Model file for the job. Use its own axes, mm. Face numbers are marked on the shaded views. A direction names the side the tool comes from. Round coordinates to 2 decimals unless told otherwise and drop trailing zeros. Loops run counter-clockwise (first coordinate to the right, second up) from the corner with the lowest first, then second, coordinate; pieces in that order, holes last. Notation, with made-up numbers: M 46,67 L 66,67 A28 cw 66,103 Z; hole C 80.5,11 d10. An arc over 180 degrees is marked long. Use a Markdown table: item, result. Add a question column.
Q1. Cut at B-B (z = -152). Give the cut face in (x, y), plus the area to 4 significant figures.
Q2. Pin check, flat tips, straight feed: pin 1 (1.9 mm diameter, centred on x = -305, z = -608, fed in from +Y); pin 2 (9 mm diameter, centred on x = -76, y = 69, fed in from -Z); pin 3 (3 mm diameter, centred on x = 179, z = -605.5, fed in from +Y); pin 4 (9 mm diameter, centred on x = 260, y = 233, fed in from +Z). Stop position of each tip, or through.
Q3. Probe line 1 (X direction, y = 49, z = -402); line 2 (Y direction, x = -209.5, z = -435); line 3 (Y direction, x = 66.5, z = -34). List the from-to ranges inside material, lowest first. Write a range as from..to.
Q4. Tool access for the marked faces 1 and 2: list every direction of +Z, -Z, +X, -X, +Y, -Y with a clear straight run to the whole face (end or side of a thin tool).
Q5. Cut at A-A (y = 185). Give the cut face in (x, z), plus the area to 3 significant figures.
Q6. Cut at C-C (x = 105). Give the cut face in (y, z).
Q7. Cut at D-D (z = -446). Give the cut face in (x, y).
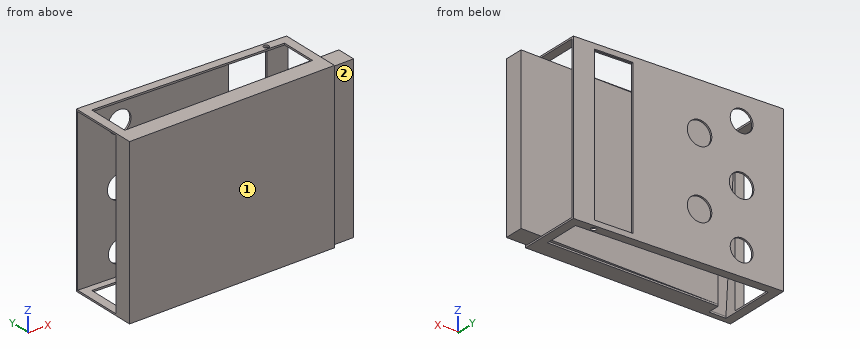
from build123d import *

# Parameters (mm, degrees)
BOSS_EXTRUDE1_DEPTH = 609.6
SHELL1_T            = -6.35
CUT_EXTRUDE1_DEPTH  = 609.6
BOSS_EXTRUDE3_DEPTH = 596.9
BOSS_EXTRUDE4_DEPTH = 95.25
SKETCH8_W           = 31.75
SKETCH8_H           = 44.45
BOSS_EXTRUDE5_DEPTH = 603.25
SKETCH9_W           = 63.5
SKETCH9_H           = 44.45
CUT_EXTRUDE2_DEPTH  = 6.35
SKETCH10_R          = 41.275
SKETCH10_R_2        = 44.45
CUT_EXTRUDE3_DEPTH  = 6.35
SKETCH12_W          = 139.7
SKETCH12_H          = 571.5
CUT_EXTRUDE4_DEPTH  = 6.35
SKETCH13_R          = 9.525
CUT_EXTRUDE5_DEPTH  = 609.6


with BuildPart() as part:
    # Sketch1 → Boss-Extrude1 (new body)
    with BuildSketch(Plane.XY):
        Polygon((-373.981578947, 0), (388.018421053, 0), (388.018421053, 228.6), (-373.981578947, 254), align=None)
    extrude(amount=-BOSS_EXTRUDE1_DEPTH)

    # Shell1
    shell1_openings = [part.faces().sort_by_distance(p)[0] for p in [
        (-373.981578947, 127, -304.8),
        (388.018421053, 114.3, -304.8),
    ]]
    offset(amount=SHELL1_T, openings=shell1_openings, kind=Kind.INTERSECTION)

    # Sketch2 → Cut-Extrude1 (cut)
    with BuildSketch(Plane.XY):
        Polygon((-342.231578947, 221.174032675), (356.268421053, 197.890699341), (356.268421053, 63.5), (-342.231578947, 63.5), align=None)
    extrude(amount=-CUT_EXTRUDE1_DEPTH, mode=Mode.SUBTRACT)

    # Sketch5 → Boss-Extrude3 (add)
    with BuildSketch(Plane.XY.offset(-603.25)):
        Polygon((-278.731578947, 63.5), (464.218421053, 76.696522884), (464.218421053, 6.35), (-278.731578947, 6.35), align=None)
    extrude(amount=BOSS_EXTRUDE3_DEPTH)

    # Sketch6 → Boss-Extrude4 (add)
    with BuildSketch(Plane.ZY.offset(278.731578947)):
        Polygon((-6.35, 63.5), (-603.25, 19.05), (-603.25, 6.35), (-6.35, 6.35), align=None)
    extrude(amount=BOSS_EXTRUDE4_DEPTH)

    # Sketch8 → Boss-Extrude5 (add)
    with BuildSketch(Plane(origin=(0, 0, -609.6), x_dir=(-1, 0, 0), z_dir=(0, 0, -1))):
        with Locations((358.106578947, 41.275)):
            Rectangle(SKETCH8_W, SKETCH8_H)
    extrude(amount=-BOSS_EXTRUDE5_DEPTH)

    # Sketch9 → Cut-Extrude2 (cut)
    with BuildSketch(Plane(origin=(0, 0, -609.6), x_dir=(-1, 0, 0), z_dir=(0, 0, -1))):
        with Locations((310.481578947, 41.275)):
            Rectangle(SKETCH9_W, SKETCH9_H)
    extrude(amount=-CUT_EXTRUDE2_DEPTH, mode=Mode.SUBTRACT)

    # Sketch10 → Cut-Extrude3 (cut)
    with BuildSketch(Plane(origin=(8.042195806, 241.265874175, 0), x_dir=(0.999444907, -0.03331483, 0), z_dir=(0.03331483, 0.999444907, 0))):
        with Locations((-229.835951262, 88.9)):
            Circle(SKETCH10_R)
        with Locations((-229.835951262, 520.7)):
            Circle(SKETCH10_R)
        with Locations((-77.435951262, 431.8)):
            Circle(SKETCH10_R_2)
        with Locations((-77.435951262, 177.8)):
            Circle(SKETCH10_R_2)
        with Locations((-229.835951262, 304.8)):
            Circle(SKETCH10_R_2)
    extrude(amount=-CUT_EXTRUDE3_DEPTH, mode=Mode.SUBTRACT)

    # Sketch12 → Cut-Extrude4 (cut)
    with BuildSketch(Plane(origin=(8.042195806, 241.265874175, 0), x_dir=(0.999444907, -0.03331483, 0), z_dir=(0.03331483, 0.999444907, 0))):
        with Locations((234.137264544, 304.8)):
            Rectangle(SKETCH12_W, SKETCH12_H)
    extrude(amount=-CUT_EXTRUDE4_DEPTH, mode=Mode.SUBTRACT)

    # Sketch13 → Cut-Extrude5 (cut)
    with BuildSketch(Plane.XY):
        with Locations((301.467767378, 213.990365252)):
            Circle(SKETCH13_R)
    extrude(amount=-CUT_EXTRUDE5_DEPTH, mode=Mode.SUBTRACT)


solid = part.part
Checked values:
| question | item | result |
|---|---|---|
| 1 | outline | M -373.98,0 L 388.02,0 L 388.02,6.35 L 464.22,6.35 L 464.22,76.7 L -278.73,63.5 L -278.73,52.65 L -342.23,52.65 L -342.23,63.5 L -373.98,63.5 Z; M -373.98,247.65 L -105.74,238.71 L -105.53,245.05 L -373.98,254 Z; M -33.39,236.29 L 172.03,229.45 L 172.24,235.79 L -33.17,242.64 Z; M 311.65,224.79 L 388.02,222.25 L 388.02,228.6 L 311.86,231.14 Z |
| 1 | area | 60,450 mm^2 |
| 2 | pin 1 | stops at y = 251.73 |
| 2 | pin 2 | stops at z = -603.25 |
| 2 | pin 3 | stops at y = 235.62 |
| 2 | pin 4 | stops at z = 0 |
| 3 | line 1 | x = -373.98..-342.23, -278.73..464.22 |
| 3 | line 2 | y = 0..64.73, 242.16..248.52 |
| 3 | line 3 | y = 0..69.63, 232.96..239.32 |
| 4 | face 1 | +Z, -Z, +X, -X, -Y |
| 4 | face 2 | +Z, -Z, +X, -Y |
| 5 | outline | M -373.98,-609.6 L -342.23,-609.6 L -342.23,-603.25 L -373.98,-603.25 Z; M -373.98,-6.35 L -342.23,-6.35 L -342.23,0 L -373.98,0 Z; M 356.27,-609.6 L 388.02,-609.6 L 388.02,-603.25 L 356.27,-603.25 Z; M 356.27,-6.35 L 388.02,-6.35 L 388.02,0 L 356.27,0 Z |
| 5 | area | 806 mm^2 |
| 6 | outline | M 0,-609.6 L 63.5,-609.6 L 63.5,-603.25 L 70.32,-603.25 L 70.32,-6.35 L 63.5,-6.35 L 63.5,0 L 0,0 Z; M 206.27,-609.6 L 238.03,-609.6 L 238.03,0 L 206.27,0 L 206.27,-6.35 L 231.68,-6.35 L 231.68,-603.25 L 206.27,-603.25 Z |
| 7 | outline | M -373.98,0 L 388.02,0 L 388.02,6.35 L 464.22,6.35 L 464.22,76.7 L -278.73,63.5 L -278.73,30.76 L -342.23,30.76 L -342.23,63.5 L -373.98,63.5 Z; M -373.98,247.65 L -111.66,238.9 L -111.45,245.25 L -373.98,254 Z; M -27.46,236.1 L 172.03,229.45 L 172.24,235.79 L -27.25,242.44 Z; M 311.65,224.79 L 388.02,222.25 L 388.02,228.6 L 311.86,231.14 Z |
